For this review, take the finished solid that the model builds, in its own axes (mm). A direction names the side the tool comes from. Round coordinates to 2 decimals unless told otherwise and drop trailing zeros. Loops run counter-clockwise (first coordinate to the right, second up) from the corner with the lowest first, then second, coordinate; pieces in that order, holes last.
1. Tool access review of faces 4 (the cylindrical face through (17.638, -0.33, -7.493)), 5 (the flat face through (17.004, -0.01, -4.991)): name each direction out of +Z, -Z, +X, -X, +Y, -Y from which nothing blocks a thin tool from reaching the whole face with its end or side.
2. Consider section A-A on y = 0. State the section outline as (x, z) points, then the cut area to 3 significant figures.
3. Draft analysis for pull direction Z (two halves, no side actions). For faces 1 (the cylindrical face through (21.147, -0.553, -2.026)), 2 (the cylindrical face through (4.93, -0.07, -1.5)), 3 (the flat face through (0, 0, 0)), state which applies: released by +Z, released by -Z, zero draft, split by the parting line, or undercut.
4. Consider section B-B on x = 11.25. State the section outline as (y, z) points.
5. Consider section D-D on y = -3. State the section outline as (x, z) points.
6. Consider section C-C on z = 4. State the section outline as (x, y) points, then the cut area to 3 significant figures.
7. To check wall thickness, follow line 1 along X through (y, z) = (-0.5, 1); line 2 along Z through (x, y) = (7.5, 0.5); line 3 along X through (y, z) = (2.25, 3.75). State the ranges of each line that lie inside material, in increasing order.
8. Clearance check with flat-ended pins moving along their axes: pin 1 Ø2 at (x, y) = (22, 1) entering from +Z; pin 2 Ø1.5 at (x, y) = (18.5, 5.5) entering from +Z; pin 3 Ø1 at (x, z) = (13.5, -2) entering from -Y. State where each tip first meets the part, or that it passes through.
from build123d import *

# Parameters (mm, degrees)
F3_DEPTH      = 7.501
F3_DEPTH_BACK = 7.501
F4_R          = 0.75
F5_DEPTH      = 10


with BuildPart() as f1:
    # F0 (on Front) → F1 (revolve)
    with BuildSketch(Plane.XZ):
        Polygon((30, 7.5), (10, 7.5), (10, 1.5), (0, 1.5), (0, 0), (30, 0), align=None)
    revolve(axis=Axis((8.7773360142, 0, 0), (1, 0, 0)))

    # F2 (on Front) → F3 (cut, two sides)
    with BuildSketch(Plane.XZ) as f3_sk:
        Polygon((21.3397459622, 7.5), (30, -7.5), (30, 7.5), align=None)
    extrude(amount=-F3_DEPTH, mode=Mode.SUBTRACT)
    extrude(f3_sk.sketch, amount=F3_DEPTH_BACK, mode=Mode.SUBTRACT)

    # F4 (on face) → F5 (cut)
    with BuildSketch(Plane(origin=(19.2524047358, 0, 11.1153810568), x_dir=(0, 1, 0), z_dir=(0.8660254038, 0, 0.5))):
        with Locations((0, -12.8349364905)):
            Circle(F4_R)
    extrude(amount=-F5_DEPTH, mode=Mode.SUBTRACT)


solid = f1.part
Resolved:
1. face 4: +X, -X
1. face 5: none
2. outline: (0, -1.5) - (10, -1.5) - (10, -7.5) - (30, -7.5) - (26.04, -0.65) - (17.38, -5.65) - (16.63, -4.35) - (25.29, 0.65) - (21.34, 7.5) - (10, 7.5) - (10, 1.5) - (0, 1.5) - close
2. area: 250 mm2
3. face 1: undercut
3. face 2: split by the parting line
3. face 3: zero draft
4. outline: circle Ø15 at (0, 0)
5. outline: (10, -6.87) - (29.64, -6.87) - (21.7, 6.87) - (10, 6.87) - close
6. outline: (10, -6.34) - (23.36, -6.34) - (23.36, 6.34) - (10, 6.34) - close
6. area: 170 mm2
7. line 1: x = 0 to 25.09
7. line 2: z = -1.41 to 1.41
7. line 3: x = 10 to 23.5
8. pin 1: stops at z = 7.5
8. pin 2: stops at z = 5.8
8. pin 3: stops at y = -7.35
